Can you work these out from the model? Positions are in its coordinate system, mm. A direction names the side the tool comes from. Round coordinates to 2 decimals unless told otherwise and drop trailing zeros. Loops run counter-clockwise (first coordinate to the right, second up) from the corner with the lowest first, then second, coordinate; pieces in that order, holes last. Notation, with made-up numbers: (-16.5, 22) -> (-10.5, 22) arc R18 cw to (-10.5, 47) -> close; hole circle Ø7 at (74, -6.75). An arc over 180 degrees is marked (long way). Use a Markdown table: item, result.
Autodesk Inventor part; units mm, degrees
ref_plane "YZ Plane" through (0, 0, 0) normal (1, 0, 0) x (0, 1, 0)
ref_plane "XZ Plane" through (0, 0, 0) normal (0, 1, 0) x (-1, 0, 0)
ref_plane "XY Plane" through (0, 0, 0) normal (0, 0, 1) x (1, 0, 0)
sketch "Sketch1" plane through (0, 0, 0) normal (1, 0, 0) x (0, 1, 0)
  line L0 (0, 14.7987) -> (0, -14.7987)
  line L1 (20.2387, -8.912) -> (20.2387, 8.912)
  line L2 (0, 14.7987) -> (20.2387, 8.912)
  line L3 (20.2387, 8.912) -> (23.2652, 8.0317)
  line L4 (23.2652, 8.0317) -> (23.2652, 10.0317)
  line L5 (23.2652, 10.0317) -> (0.8483, 16.552)
  arc A0 (10.1758, 29.9776) -> (0, 14.7987) centre (53.1668, -9.8435) ccw
  line L6 (0, 0) -> (4.1623, 0)
  dimension "d0" = 2
  dimension "d1" = 23.3459
  dimension "d2" = 58.5999
  dimension "d3" = 29.5974
  dimension "d4" = 20.2387
  dimension "d5" = 17.8241
  dimension "d6" = 1.7533
revolve "Revolution1" add sketch "Sketch1" angle 360 about axis through (0, 0, 0) along (0, 1, 0)
sketch "Sketch2" plane through (0, 0, 0) normal (1, 0, 0) x (0, 1, 0)
  arc A0 (10.1596, 29.9776) -> (0.8483, 16.552) centre (53.1862, -9.8051) ccw
  line L0 (0.8483, 16.552) -> (23.2652, 10.0317)
  line L1 (23.2652, 9.4492) -> (23.2652, 16.4492)
  line L2 (10.1596, 29.9776) -> (23.2652, 16.4492)
  line L3 (0.8483, -16.552) -> (23.2652, -10.0317)
  line L4 (0.8483, 16.552) -> (23.2652, 10.0317)
  line L5 (10.5533, 26.4347) -> (20.7474, 17.0064)
  line L6 (7.1516, 20.973) -> (10.5533, 26.4347)
  line L7 (7.1516, 20.973) -> (20.7474, 14.6029)
  line L8 (20.7474, 17.0064) -> (20.7474, 14.6029)
  line L9 (23.2652, 9.4492) -> (0.7694, 16.1344)
  line L10 (0.7694, 16.1344) -> (0.8483, 16.552)
  point P0 (0, 0)
  dimension "d8" = 18.8355
  dimension "d9" = 22.4169
  dimension "d10" = 7
  dimension "d11" = 58.5999
  dimension "d12" = 23.3459
  dimension "d15" = 13.4256
extrude "Extrusion1" add sketch "Sketch2" along normal mid plane 3
fillet "Fillet1" radius 1 4 edges at (0, 10.5533, 26.4347) (0, 7.1516, 20.973) (0, 20.7474, 17.0064) (0, 20.7474, 14.6029)
pattern_circular "Circular Pattern1" count 6 over 360 about axis through (0, 11.6326, 0) along (0, 1, 0) of "Extrusion1"
properties part number "Internal Structure"
1. Will these pins go through, and if not, where does the flat tip stop? pin 1 Ø1.8 at (x, z) = (13.5, 8.5) entering from -Y; pin 2 Ø3 at (y, z) = (13.5, -9.5) entering from +X; pin 3 Ø5 at (x, z) = (5.5, 19.5) entering from +Y; pin 4 Ø1.8 at (x, z) = (13.5, -9) entering from -Y.
Answer sheet:
| item | result |
|---|---|
| pin 1 | stops at y = 0.12 |
| pin 2 | stops at x = 22.05 |
| pin 3 | passes through |
| pin 4 | stops at y = 0.25 |
2. I want a section at B-B (y = 4.25). Please give me the cut outline in (x, z), plus the area to 3 significant figures.
Answer sheet:
| item | result |
|---|---|
| outline | (-20.18, -9.92) -> (-18.68, -12.51) -> (-12.66, -9.04) arc R15.56 ccw to (-1.5, -15.49) -> (-1.5, -22.43) -> (1.5, -22.43) -> (1.5, -15.49) arc R15.56 ccw to (12.66, -9.04) -> (18.68, -12.51) -> (20.18, -9.92) -> (14.16, -6.45) arc R15.56 ccw to (14.16, 6.45) -> (20.18, 9.92) -> (18.68, 12.51) -> (12.66, 9.04) arc R15.56 ccw to (1.5, 15.49) -> (1.5, 22.43) -> (-1.5, 22.43) -> (-1.5, 15.49) arc R15.56 ccw to (-12.66, 9.04) -> (-18.68, 12.51) -> (-20.18, 9.92) -> (-14.16, 6.45) arc R15.56 ccw to (-14.16, -6.45) -> close; hole circle Ø27.13 at (0, 0) |
| area | 307 mm² |
3. I need wall thicknesses on line 1 (X direction, y = 21, z = -9); line 2 (X direction, y = 8.25, z = 17); line 3 (X direction, y = 9.5, z = 0). Which ranges of each line are inside material? Lowest first, please.
Answer sheet:
| item | result |
|---|---|
| line 1 | x = -16.5 to -12.59, -5.77 to 5.77, 12.59 to 16.5 |
| line 2 | x = -1.5 to 1.5 |
| line 3 | x = -14.04 to -12.04, 12.04 to 14.04 |
4. I want a section at A-A (z = -23). Please give me the cut outline in (x, y), plus the area to 3 significant figures.
Answer sheet:
| item | result |
|---|---|
| outline | (-1.5, 4.63) -> (1.5, 4.63) -> (1.5, 8.41) -> (-1.5, 8.41) -> close; (-1.5, 14.27) -> (1.5, 14.27) -> (1.5, 16.92) -> (-1.5, 16.92) -> close |
| area | 19.3 mm² |
5. If we mould it in two halves opening along X, with no side actions, what happens to faces 1 (the flat face through (20.51, 8.83, -11.81)), 2 (the flat face through (15.433, 13.854, 8.934)), 3 (the conical face through (-13.337, 11.9, 0.081)), 4 (the flat face through (-0.02, 16.62, 23.31))? For each: +X half, -X half, draft (parallel to the pull), parting line (faces both ways), or undercut.
Answer sheet:
| item | result |
|---|---|
| face 1 | undercut |
| face 2 | undercut |
| face 3 | -X half |
| face 4 | draft |
6. I want a section at C-C (y = 15). State how many separate pieces and enclosed holes the cut face has, plus the area to 3 significant figures.
Answer sheet:
| item | result |
|---|---|
| separate pieces | 7 |
| enclosed holes | 1 |
| area | 280 mm² |
7. Which directions (+Z, -Z, +X, -X, +Y, -Y) give clear straight access to the entire face, cutting with the end or side of a thin tool? Please do faces 5 (the cylindrical face through (-20.36, 4.97, 11.73)), 6 (the flat face through (-0.02, 15.87, 21.52)), 7 (the flat face through (-14, 20.747, -8)).
Answer sheet:
| item | result |
|---|---|
| face 5 | +Z, -X, -Y |
| face 6 | +X, -X |
| face 7 | none |
